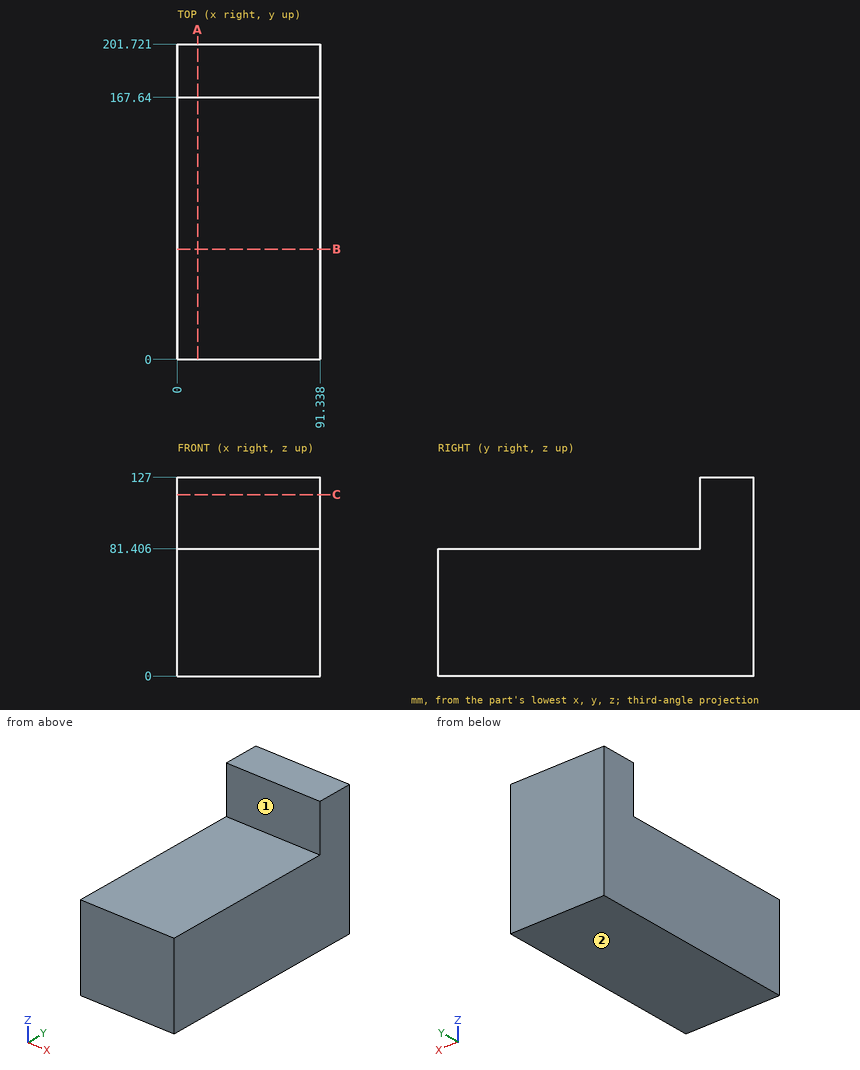
For this review, use the dimensioned drawing (mm, ordinates from the lowest corner) and the shaded views. A direction names the side the tool comes from. Give positions to 0.01 mm unless a question says otherwise; leave off trailing zeros. Loops run counter-clockwise (first coordinate to the right, second up) from the corner with the lowest first, then second, coordinate; pieces in that order, holes last. Notation, with made-up numbers: (8.5, 83) -> (65.5, 83) arc R18 cw to (65.5, 99) -> close; hole circle Ø2 at (-16, 43). An arc over 180 degrees is marked (long way). Use CSV: the item, a comma, the result in double quotes.
1. To check wall thickness, follow probe 1 along Z at (x, y) = (85.5, 121.5); probe 2 along Y at (x, z) = (54, 110.5). State the ranges of each line that lie inside material, in increasing order. Write a range as from..to.
Result:
probe 1,"z = 0..81.41"
probe 2,"y = 167.64..201.72"
2. For P1, Ø3, axis at x = 17, z = 57.5, coming from the -Y side; P2, Ø2, axis at x = 33.5, y = 155.5, coming from the +Z side, all flat-tipped, find the tip position at first contact; note any pin that passes through.
Result:
P1,"stops at y = 0"
P2,"stops at z = 81.41"
3. Machinability: for the marked faces 1 and 2, which of the approach directions +Z, -Z, +X, -X, +Y, -Y give a long, thin tool a straight path to every point of the face, cutting with its end or side? Answer none if there is none.
Result:
face 1,"+Z, +X, -X, -Y"
face 2,"-Z, +X, -X, +Y, -Y"
4. Consider section C-C, the plane z = 116. Write out the cut boundary in (x, y), then the cut area to 3 significant figures.
Result:
outline,"(0, 167.64) -> (91.34, 167.64) -> (91.34, 201.72) -> (0, 201.72) -> close"
area,"3,110 mm²"
5. Consider section B-B, the plane y = 70.5. Write out the cut boundary in (x, z), then the cut area to 3 significant figures.
Result:
outline,"(0, 0) -> (91.34, 0) -> (91.34, 81.41) -> (0, 81.41) -> close"
area,"7,440 mm²"
6. Consider section A-A, the plane x = 13. Write out the cut boundary in (y, z), then the cut area to 3 significant figures.
Result:
outline,"(0, 0) -> (201.72, 0) -> (201.72, 127) -> (167.64, 127) -> (167.64, 81.41) -> (0, 81.41) -> close"
area,"18,000 mm²"
